Autodesk Inventor part; units mm, degrees
ref_plane "YZ Plane" through (0, 0, 0) normal (1, 0, 0) x (0, 1, 0)
ref_plane "XZ Plane" through (0, 0, 0) normal (0, 1, 0) x (-1, 0, 0)
ref_plane "XY Plane" through (0, 0, 0) normal (0, 0, 1) x (1, 0, 0)
sketch "Sketch1" plane through (0, 0, 0) normal (0, 0, 1) x (1, 0, 0)
  line L0 (0, -50.8) -> (0, 50.8)
  line L1 (0, 50.8) -> (6.35, 50.8)
  line L2 (6.35, 50.8) -> (6.35, 6.35)
  line L3 (6.35, 6.35) -> (57.15, 6.35)
  line L4 (57.15, 6.35) -> (57.15, -6.35)
  line L5 (57.15, -6.35) -> (6.35, -6.35)
  line L6 (6.35, -6.35) -> (6.35, -50.8)
  line L7 (6.35, -50.8) -> (0, -50.8)
  line L8 (0, 0) -> (57.15, 0) construction
  dimension "d0" = 12.7
  dimension "d1" = 101.6
  dimension "d2" = 50.8
  dimension "d3" = 6.35
extrude "Extrusion1" add sketch "Sketch1" along normal mid plane 50.8
fillet "Fillet1" radius 25.4 6 edges at (57.15, 0, 25.4) (57.15, 0, -25.4) (3.175, 50.8, -25.4) (3.175, 50.8, 25.4) (3.175, -50.8, 25.4) (3.175, -50.8, -25.4)
fillet "Fillet2" radius 3.175 12 edges at (49.7105, 6.35, 17.9605) (19.05, 6.35, -25.4) (19.05, 6.35, 25.4) (49.7105, -6.35, 17.9605) (19.05, -6.35, -25.4) (19.05, -6.35, 25.4) (6.35, 15.875, -25.4) (6.35, 15.875, 25.4) (6.35, 43.3605, -17.9605) (6.35, -15.875, 25.4) (6.35, -15.875, -25.4) (6.35, -43.3605, 17.9605)
hole "Hole1" at (31.75, 6.35, 0) direction (0, -1, 0) diameter 19.05 end through all
sketch "Sketch2" plane through (6.35, 6.35, 22.225) normal (1, 0, 0) x (0, 0, -1)
  line L0 (22.225, 19.05) -> (22.225, -31.75) construction
  point P0 (22.225, -6.35)
  point P1 (22.225, -6.35)
  dimension "d17" = 50.8
hole "Hole2" at (6.35, 25.4, 0) at (6.35, -25.4, 0) direction (-1, 0, 0) diameter 10.5918 end through all
properties part number "Door Hinge" material "Steel, Alloy"
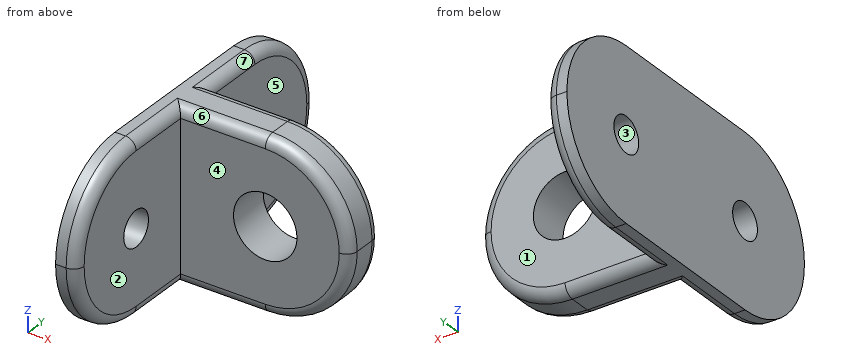
Geometry check sheet. Reference: the model listing, model coordinates, mm. Face numbers are marked on the shaded views. A direction names the side the tool comes from. Coordinates: 2 decimals unless noted, no trailing zeros. Order: outer loops, then holes, each group sorted by start corner. A loop starts at its lowest first (then second) coordinate and runs counter-clockwise, first axis right, second up.
Item 1: Section check B-B (y = 14.5). Enter the section's corners in (x, z) (3 decimals), plus the area to 3 significant figures.
Item 2: Mould release check, pull along Y, two halves, no side actions. Record for the marked faces 1, 2 and 3: released by +Y, released by -Y, zero draft, split by the parting line, or undercut.
Item 3: Section check A-A (x = 25). Enter the section's corners in (y, z) (3 decimals), plus the area to 3 significant figures.
Item 4: Scan lines: line 1 along Y through (x, z) = (2.5, 0); line 2 along Z through (x, y) = (2, 25); line 3 along Y through (x, z) = (4, 0). Record each from-to range of solid material in increasing order.
Item 5: Depth check by flat-ended pin: pin 1 (2 mm diameter, centred on x = 8.5, z = -2.5, fed in from -Y); pin 2 (1.5 mm diameter, centred on y = 39, z = 8, fed in from +X); pin 3 (12 mm diameter, centred on x = 48, z = -15, fed in from +Y). Enter the tip coordinate at first touch or a pass-through.
Item 6: Tool access check on the marked faces 4, 5, 6 and 7. Record the directions out of +Z, -Z, +X, -X, +Y, -Y that give a thin tool (end or side, any length) a straight path to the whole face; none if there is none.
Check sheet entries:
1. outline: (0, -25.4) - (3.175, -25.4) arc R3.175 ccw to (6.35, -22.225) - (6.35, 22.225) arc R3.175 ccw to (3.175, 25.4) - (0, 25.4) - close
1. area: 318 mm2
2. face 1: released by +Y
2. face 2: zero draft
2. face 3: undercut
3. outline: (-6.35, -22.225) arc R3.175 ccw to (-3.175, -25.4) - (3.175, -25.4) arc R3.175 ccw to (6.35, -22.225) - (6.35, -6.72) - (-6.35, -6.72) - close; (-6.35, 6.72) - (6.35, 6.72) - (6.35, 22.225) arc R3.175 ccw to (3.175, 25.4) - (-3.175, 25.4) arc R3.175 ccw to (-6.35, 22.225) - close
3. area: 466 mm2
4. line 1: y = -50.8 to -30.7, -20.1 to 20.1, 30.7 to 50.8
4. line 2: z = -25.4 to -5.28, 5.28 to 25.4
4. line 3: y = -50.69 to -30.7, -20.1 to 20.1, 30.7 to 50.69
5. pin 1: stops at y = -6.35
5. pin 2: stops at x = 6.35
5. pin 3: stops at y = 6.35
6. face 4: +Z, -Z, +X, -Y
6. face 5: +Z, -Z, +X, +Y
6. face 6: +Z, +X, -Y
6. face 7: +Z, +X, +Y
